Input: part model. Units: mm. Frame: model coordinates. A direction names the side the tool comes from. Give positions to 0.01 mm unless a question says otherwise; leave off trailing zeros. Write each loop counter-clockwise with the first axis right and the second up, starting at its lowest first coordinate (ties: lowest second). Pieces come first, ordered by that corner, then holes. Notation, with made-up numbers: (13.25, 81.5) -> (62.25, 81.5) arc R24 cw to (62.25, 93.5) -> close; hole circle Ø5 at (81.5, 74). An arc over 180 degrees is marked (long way). Answer as a JSON object with one key per item and string values. Group by question number.
Autodesk Inventor part; units mm, degrees
ref_plane "YZ Plane" through (0, 0, 0) normal (1, 0, 0) x (0, 1, 0)
ref_plane "XZ Plane" through (0, 0, 0) normal (0, 1, 0) x (-1, 0, 0)
ref_plane "XY Plane" through (0, 0, 0) normal (0, 0, 1) x (1, 0, 0)
sketch "Sketch1" plane through (0, 0, 0) normal (1, 0, 0) x (0, 1, 0)
  line L0 (-20, 18) -> (20, 18)
  line L1 (20, 18) -> (20, -18)
  line L2 (20, -18) -> (-20, -18)
  line L3 (-20, -18) -> (-20, 18)
  line L4 (-20, 18) -> (20, -18) construction
  line L5 (20, 18) -> (-20, -18) construction
  circle A0 centre (8, 13) radius 1.75
  circle A1 centre (8, -13) radius 1.75
  line L6 (20, 0) -> (-20, 0) construction
  line L7 (0, 18) -> (0, -18) construction
  circle A2 centre (16, 6) radius 1.75
  circle A3 centre (16, -6) radius 1.75
  circle A4 centre (-8, 13) radius 1.75
  circle A5 centre (-8, -13) radius 1.75
  circle A6 centre (-16, 6) radius 1.75
  circle A7 centre (-16, -6) radius 1.75
  point P0 (0, 0)
  dimension "d0" = 40
  dimension "d1" = 36
  dimension "d2" = 3.5
  dimension "d3" = 3.5
  dimension "d4" = 13
  dimension "d5" = 13
  dimension "d6" = 8
  dimension "d7" = 8
  dimension "d8" = 3.5
  dimension "d9" = 4
  dimension "d10" = 6
  dimension "d11" = 3.5
  dimension "d12" = 6
  dimension "d13" = 4
extrude "Extrusion1" add sketch "Sketch1" along normal blind 5
sketch "Sketch2" plane through (5, 0, 0) normal (1, 0, 0) x (0, 0, -1)
  circle A0 centre (-13, 8) radius 1.75 construction
  line L0 (-13, 9.75) -> (-13, 8) construction
  circle A1 centre (-13, 8) radius 3
  circle A2 centre (-6, 16) radius 1.75 construction
  line L1 (-6, 17.75) -> (-6, 16) construction
  circle A3 centre (6, 16) radius 1.75 construction
  line L2 (-6, 16) -> (6, 16) construction
  circle A4 centre (13, 8) radius 1.75 construction
  line L3 (6, 16) -> (13, 8) construction
  circle A5 centre (-6, 16) radius 3
  circle A6 centre (6, 16) radius 3
  circle A7 centre (13, 8) radius 3
  line L4 (-18, 20) -> (-18, -20) construction
  line L5 (-18, 0) -> (18, 0) construction
  line L6 (18, 20) -> (18, -20) construction
  circle A8 centre (-13, -8) radius 3
  circle A9 centre (-6, -16) radius 3
  circle A10 centre (6, -16) radius 3
  circle A11 centre (13, -8) radius 3
  point P0 (0, 0)
  dimension "d16" = 6
  dimension "d17" = 6
  dimension "d18" = 6
  dimension "d19" = 6
extrude "Extrusion2" cut sketch "Sketch2" against normal blind 3
sketch "Sketch3" plane through (5, 0, 0) normal (1, 0, 0) x (0, 0, -1)
  circle A0 centre (-12.96, -16) radius 1.5
  circle A1 centre (12.96, -16) radius 1.5
  line L0 (0, 0) -> (0, -23.2613) construction
  line L1 (-18, -20) -> (18, -20) construction
  dimension "d22" = 3
  dimension "d23" = 3
  dimension "d24" = 12.96
  dimension "d25" = 12.96
  dimension "d26" = 4
  dimension "d27" = 4
extrude "Extrusion3" cut sketch "Sketch3" against normal blind 5
properties part number "Steam Chest Cover" material "Iron, Cast"
1. Reachability of faces 1 (the face through (1, -7.1, -14.5)), 2 (the face through (2, -8, -15)) from +Z, -Z, +X, -X, +Y, -Y: full face, straight path, thin tool, end or side. Return the list, or none.
2. Mould query, pull axis Y, two halves, no side actions, for faces 3 (the face through (2, -20, 0)), 4 (the face through (2, 0, 18)), 5 (the face through (3.52, 13.07, -5.35)). Classes: pulls with the +Y half, pulls with the -Y half, needs draft (parallel to the pull), parting line crosses it, or undercut.
3. Section B-B (x = 2.6). State how many separate pieces and enclosed holes the cut face has, plus the area to 3 significant figures.
4. Section D-D (y = 16). Return the cut outline in (x, z), plus the area to 3 significant figures.
5. Line query: line 1 (Z direction, x = 1.2, y = -8); line 2 (Y direction, x = 0.65, z = -13); line 3 (Y direction, x = 3.6, z = -13). Output: solid intervals per line, ascending.
6. Section A-A (y = -16). Return the cut outline in (x, z).
7. Section C-C (z = -7). Return the cut outline in (x, y).
8. Contact query for flat-ended pins moving along their axis: pin 1 Ø5.5 at (y, z) = (8, -13) entering from -X; pin 2 Ø5 at (y, z) = (16, -6) entering from +X; pin 3 Ø3 at (y, z) = (-8, -13) entering from -X. Output: stop coordinate, or through.
Working result:
{
 "1": {"face 1": "+X, -X", "face 2": "+X"},
 "2": {"face 3": "pulls with the -Y half", "face 4": "needs draft", "face 5": "undercut"},
 "3": {"separate pieces": "1", "enclosed holes": "10", "area": "1,200 mm^2"},
 "4": {"outline": "(0, -18) -> (5, -18) -> (5, -9) -> (2, -9) -> (2, -7.75) -> (0, -7.75) -> close; (0, -4.25) -> (2, -4.25) -> (2, -3) -> (5, -3) -> (5, 3) -> (2, 3) -> (2, 4.25) -> (0, 4.25) -> close; (0, 7.75) -> (2, 7.75) -> (2, 9) -> (5, 9) -> (5, 18) -> (0, 18) -> close", "area": "130 mm^2"},
 "5": {"line 1": "z = -18 to -14.75, -11.25 to 11.25, 14.75 to 18", "line 2": "y = -20 to -17.5, -14.5 to -9.75, -6.25 to 6.25, 9.75 to 20", "line 3": "y = -20 to -17.5, -14.5 to -11, -5 to 5, 11 to 20"},
 "6": {"outline": "(0, -18) -> (5, -18) -> (5, -14.46) -> (0, -14.46) -> close; (0, -11.46) -> (5, -11.46) -> (5, -9) -> (2, -9) -> (2, -7.75) -> (0, -7.75) -> close; (0, -4.25) -> (2, -4.25) -> (2, -3) -> (5, -3) -> (5, 3) -> (2, 3) -> (2, 4.25) -> (0, 4.25) -> close; (0, 7.75) -> (2, 7.75) -> (2, 9) -> (5, 9) -> (5, 11.46) -> (0, 11.46) -> close; (0, 14.46) -> (5, 14.46) -> (5, 18) -> (0, 18) -> close"},
 "7": {"outline": "(0, -20) -> (5, -20) -> (5, -18.83) -> (2, -18.83) -> (2, -17.44) -> (0, -17.44) -> close; (0, -14.56) -> (2, -14.56) -> (2, -13.17) -> (5, -13.17) -> (5, 13.17) -> (2, 13.17) -> (2, 14.56) -> (0, 14.56) -> close; (0, 17.44) -> (2, 17.44) -> (2, 18.83) -> (5, 18.83) -> (5, 20) -> (0, 20) -> close"},
 "8": {"pin 1": "stops at x = 0", "pin 2": "stops at x = 2", "pin 3": "passes through"}
}
